from build123d import *

# Parameters (mm, degrees)
BOSS_EXTRUDE1_DEPTH     = 6.35
FILLET1_R               = 3.175
CUT_EXTRUDE1_DEPTH      = 40.144028919
CUT_EXTRUDE1_DEPTH_BACK = 40.144028919
SKETCH2_R               = 1.5875
SKETCH3_R               = 3.175
BOSS_EXTRUDE2_DEPTH     = 12.7


with BuildPart() as part:
    # Sketch1 → Boss-Extrude1 (new body)
    with BuildSketch(Plane.XY):
        Polygon((3.175, 0), (6.35, 0), (6.35, 38.1), (-6.35, 38.1), (-6.35, 0), (-3.175, 0), (-3.175, 12.7), (3.175, 12.7), align=None)
    extrude(amount=BOSS_EXTRUDE1_DEPTH)

    # Fillet1
    fillet1_edges = [part.edges().sort_by_distance(p)[0] for p in [
        (-4.7625, 0, 0),
        (-4.7625, 0, 6.35),
        (4.7625, 0, 0),
        (4.7625, 0, 6.35),
    ]]
    fillet(fillet1_edges, radius=FILLET1_R - 0.0001)  # a hair under: the kernel refuses the full size

    # Sketch2 → Cut-Extrude1 (cut, two sides: drawn at the far end of the back side and taken through both)
    with BuildSketch(Plane(origin=(0, 0, 0), x_dir=(0, 0, -1), z_dir=(1, 0, 0)).offset(-CUT_EXTRUDE1_DEPTH_BACK)):
        with Locations((-3.175, 3.175)):
            Circle(SKETCH2_R)
    extrude(amount=CUT_EXTRUDE1_DEPTH + CUT_EXTRUDE1_DEPTH_BACK, mode=Mode.SUBTRACT)

    # Sketch3 → Boss-Extrude2 (add)
    with BuildSketch(Plane.XY.offset(6.35)):
        with Locations(Location((0, 31.75, 0), (0, 0, 180))):
            Circle(SKETCH3_R)
    extrude(amount=BOSS_EXTRUDE2_DEPTH)


solid = part.part
Could you check a few things on this model? Use its own coordinates, in mm. A direction names the side the tool comes from. Give positions to 0.01 mm unless a question says otherwise; leave off trailing zeros. Order: outer loops, then holes, each group sorted by start corner. A loop starts at its lowest first (then second) coordinate and runs counter-clockwise, first axis right, second up. Notation, with made-up numbers: (73, -16.5) - (101, -16.5) arc R30 ccw to (101, 5.5) - close; hole circle Ø6 at (54.5, -18). An arc over 180 degrees is marked (long way). One line per item, written item: value. Start each with the question number.
1. Imagine slicing it at D-D on y = 31.75. List the corners of the cut face in (x, z) for me (3 decimals).
2. Thinking about a two-plate mould opening in Y: for faces 1 (the face through (-6.35, 19, 3)), 2 (the face through (0, 38.1, 3)), 3 (the face through (4.7, 4.5, 2.3)), which applies, +Y half, -Y half, draft (parallel to the pull), parting line (faces both ways), or undercut?
3. Imagine slicing it at A-A on y = 11.5. List the corners of the cut face in (x, z) for me (3 decimals), plus the area to 3 significant figures.
4. For P1, Ø2, axis at x = -2, z = 8, coming from the +Y side; P2, Ø3, axis at x = -2, z = 10, coming from the -Y side; P3, Ø5, axis at y = 24, z = 9.5, coming from the -X side; P4, Ø5, axis at x = -0.5, z = 4, coming from the -Y side, each with a flat end and sliding along its axis, tell me the tip position at first contact or that it passes through.
5. If I drill on probe 1 along Z at (x, y) = (-5.25, 26); probe 2 along Y at (x, z) = (1.75, 3.5); probe 3 along Y at (x, z) = (-3.75, 4.5), over which ranges is the centre line in solid material (lowest first)?
6. Imagine slicing it at C-C on z = 2.75. List the corners of the cut face in (x, y) for me (3 decimals).
7. For faces 4 (the face through (0.69, 34.85, 12.61)), 5 (the face through (-4.74, 0.91, 5.4)), 6 (the face through (0, 12.7, 3)), which set-ups out of +Z, -Z, +X, -X, +Y, -Y let a thin tool reach every point of the face, with its end or its side?
Values:
1. outline: (-6.35, 0) - (6.35, 0) - (6.35, 6.35) - (3.175, 6.35) - (3.175, 19.05) - (-3.175, 19.05) - (-3.175, 6.35) - (-6.35, 6.35) - close
2. face 1: draft
2. face 2: +Y half
2. face 3: undercut
3. outline: (-6.35, 0) - (-3.175, 0) - (-3.175, 6.35) - (-6.35, 6.35) - close; (3.175, 0) - (6.35, 0) - (6.35, 6.35) - (3.175, 6.35) - close
3. area: 40.3 mm²
4. P1: y = 34.76
4. P2: y = 28.61
4. P3: through
4. P4: y = 12.7
5. probe 1: 0 to 6.35
5. probe 2: 12.7 to 38.1
5. probe 3: 0.29 to 2.3, 4.05 to 38.1
6. outline: (-6.35, 0.029) - (-3.175, 0.029) - (-3.175, 1.645) - (-6.35, 1.645) - close; (-6.35, 4.705) - (-3.175, 4.705) - (-3.175, 12.7) - (3.175, 12.7) - (3.175, 4.705) - (6.35, 4.705) - (6.35, 38.1) - (-6.35, 38.1) - close; (3.175, 0.029) - (6.35, 0.029) - (6.35, 1.645) - (3.175, 1.645) - close
7. face 4: +Z
7. face 5: +Z, +X, -X, -Y
7. face 6: +Z, -Z, -Y
